The listing builds one solid part. Answer for the finished solid, in the listing's coordinates (mm). Coordinates: 2 decimals unless noted, no trailing zeros. Order: outer loops, then holes, each group sorted by start corner. A loop starts at its lowest first (then second) coordinate and runs counter-clockwise, first axis right, second up. Notation, with made-up numbers: (69.25, 62) -> (101.25, 62) arc R29 cw to (101.25, 85) -> close; hole circle Ø9 at (21, 45). An arc over 180 degrees is marked (long way). Answer in a Markdown table with one row per item.
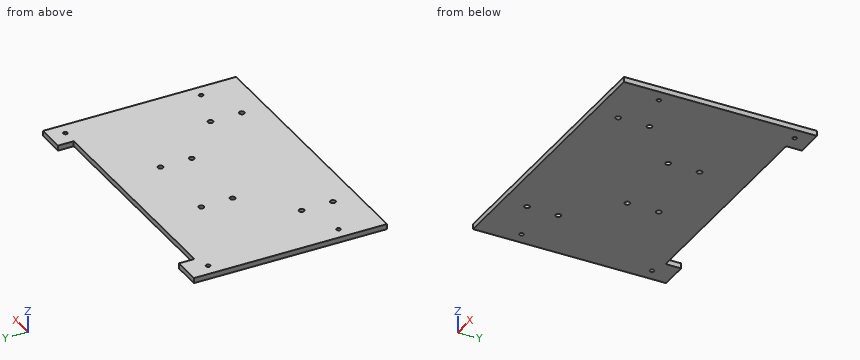
```python
from build123d import *

# Parameters (mm, degrees)
BOSS_EXTRU_1_DEPTH      = 5
ESQUISSE2_R             = 2
ENL_V_MAT_EXTRU_1_DEPTH = 169.07736314
SKETCH1_R               = 2.5
CUT_EXTRUDE1_DEPTH      = 169.07736314
SKETCH2_R               = 2.5
CUT_EXTRUDE2_DEPTH      = 24


with BuildPart() as part:
    # Esquisse1 → Boss.-Extru.1 (new body)
    with BuildSketch(Plane.XY):
        Polygon((-135, 85), (-135, 100), (-108, 100), (-108, 85), (108, 85), (108, 100), (135, 100), (135, 85), (135, -85), (-135, -85), align=None)
    extrude(amount=BOSS_EXTRU_1_DEPTH)

    # Esquisse2 → Enlèv. mat.-Extru.1 (cut, through all)
    with BuildSketch(Plane.XY.offset(5)):
        with Locations((-123, -45)):
            Circle(ESQUISSE2_R)
        with Locations((-123, 80)):
            Circle(ESQUISSE2_R)
        with Locations((123, -45)):
            Circle(ESQUISSE2_R)
        with Locations((123, 85)):
            Circle(ESQUISSE2_R)
    extrude(amount=-ENL_V_MAT_EXTRU_1_DEPTH, mode=Mode.SUBTRACT)

    # Sketch1 → Cut-Extrude1 (cut, through all)
    with BuildSketch(Plane.XY.offset(5)):
        with Locations((81.5, -31.885578019)):
            Circle(SKETCH1_R)
        with Locations((81.5, -61.885578019)):
            Circle(SKETCH1_R)
        with Locations((-81.5, -61.885578019)):
            Circle(SKETCH1_R)
        with Locations((-81.5, -31.885578019)):
            Circle(SKETCH1_R)
    extrude(amount=-CUT_EXTRUDE1_DEPTH, mode=Mode.SUBTRACT)

    # Sketch2 → Cut-Extrude2 (cut)
    with BuildSketch(Plane.XY.offset(5)):
        with Locations((36.5, 40.213230892)):
            Circle(SKETCH2_R)
        with Locations((36.5, 10.213230892)):
            Circle(SKETCH2_R)
        with Locations((-36.5, 10.213230892)):
            Circle(SKETCH2_R)
        with Locations((-36.5, 40.213230892)):
            Circle(SKETCH2_R)
    extrude(amount=-CUT_EXTRUDE2_DEPTH, mode=Mode.SUBTRACT)


solid = part.part
```
(1) Find the intervals of material crossed by line 1 along Y through (x, z) = (-81.5, 3.95); line 2 along Y through (x, z) = (36.5, 2.7); line 3 along X through (y, z) = (-33, 0.35), in increasing order. Write a range as from..to.
Check values:
| item | result |
|---|---|
| line 1 | -85..-64.39, -59.39..-34.39, -29.39..85 |
| line 2 | -85..7.71, 12.71..37.71, 42.71..85 |
| line 3 | -135..-83.74, -79.26..79.26, 83.74..135 |
(2) A flat-ended cylindrical pin translates along its axis: pin 1 (4 mm diameter, centred on x = 81.5, y = -31.89, fed in from +Z) (3 decimals). Find the tip coordinate at first contact, or state that the pin passes through.
Check values:
| item | result |
|---|---|
| pin 1 | through |
(3) A cutting plane is placed at B-B, the plane x = 18. Determine the outline of the cut face in (y, z).
Check values:
| item | result |
|---|---|
| outline | (-85, 0) -> (85, 0) -> (85, 5) -> (-85, 5) -> close |
(4) A cutting plane is placed at A-A, the plane z = 2.2. Count the separate pieces of the cut face and the enclosed holes in it, then the cut area to 3 significant figures.
Check values:
| item | result |
|---|---|
| separate pieces | 1 |
| enclosed holes | 12 |
| area | 46,500 mm² |
